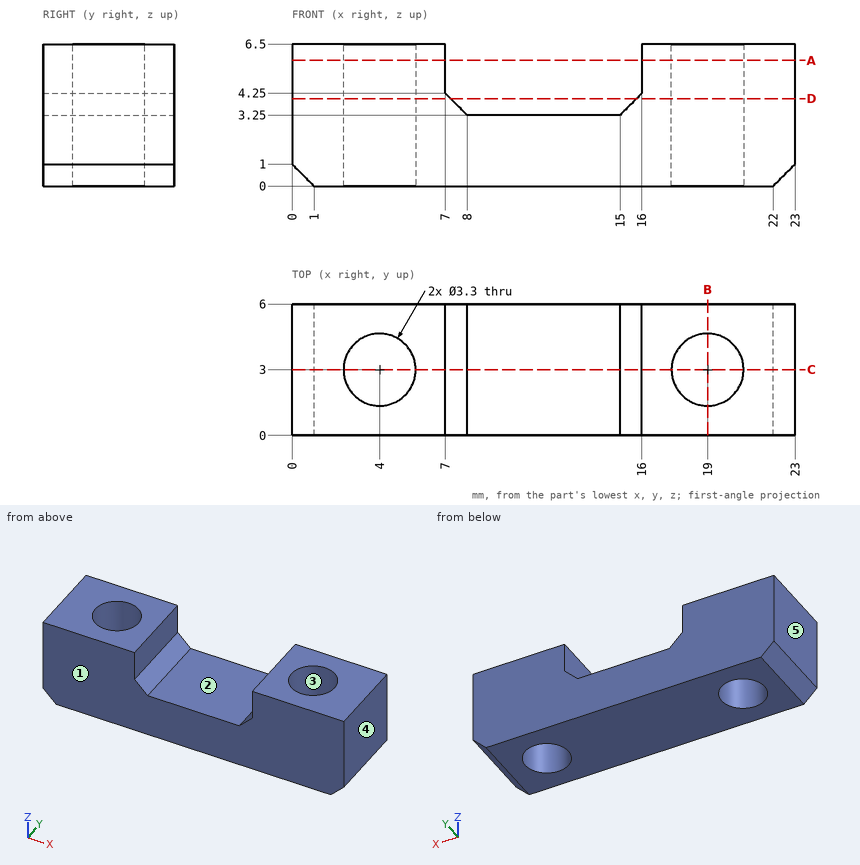
Verification items for this drawing (mm, ordinates from the low corner). A direction names the side the tool comes from. Coordinates: 2 decimals unless noted, no trailing zeros. Loops run counter-clockwise (first coordinate to the right, second up) from the corner with the lowest first, then second, coordinate; pieces in that order, holes last. Notation, with made-up numbers: (-13, -37.75) - (46, -37.75) arc R13 cw to (46, -28.75) - close; hole circle Ø7 at (7, -6.75). An arc over 180 degrees is marked (long way). Use one line per item in the form item = value. Start each with the question number.
Item 1: Gauge pin test, flat end, axial feed: pin 1 (3 mm diameter, centred on x = 11, y = 1.5, fed in from +Z). Record the tip position at first contact, or that the pin passes through.
Item 2: Thickness scan on probe 1 along Y at (x, z) = (4, 3.25); probe 2 along X at (y, z) = (3.55, 1.5); probe 3 along X at (y, z) = (1.8, 3.75). Record the ranges inside material, lowest first.
Item 3: Section check D-D, the plane z = 4. Enter the section's corners in (x, y).
Item 4: Section check B-B, the plane x = 19. Enter the section's corners in (y, z).
Item 5: Tool access check on the marked faces 1 and 2. Record the directions out of +Z, -Z, +X, -X, +Y, -Y that give a thin tool (end or side, any length) a straight path to the whole face; none if there is none.
Item 6: Mould release check, pull along X, two halves, no side actions. Record for the marked faces 3, 4 and 5: +X half, -X half, draft (parallel to the pull), parting line (faces both ways), or undercut.
Item 7: Section check A-A, the plane z = 5.75. Enter the section's corners in (x, y), and give its area (3 significant figures).
Item 8: Section check C-C, the plane y = 3. Enter the section's corners in (x, z), and give its area (4 significant figures).
Computed:
q1.pin_1 = 3.25
q2.probe_1 = 0 to 1.35, 4.65 to 6
q2.probe_2 = 0 to 2.44, 5.56 to 17.44, 20.56 to 23
q2.probe_3 = 0 to 2.87, 5.13 to 7.5, 15.5 to 17.87, 20.13 to 23
q3.outline = (0, 0) - (7.25, 0) - (7.25, 6) - (0, 6) - close; (15.75, 0) - (23, 0) - (23, 6) - (15.75, 6) - close; hole circle Ø3.3 at (4, 3); hole circle Ø3.3 at (19, 3)
q4.outline = (0, 0) - (1.35, 0) - (1.35, 6.5) - (0, 6.5) - close; (4.65, 0) - (6, 0) - (6, 6.5) - (4.65, 6.5) - close
q5.face_1 = +Z, -Z, +X, -X, -Y
q5.face_2 = +Z, +Y, -Y
q6.face_3 = undercut
q6.face_4 = +X half
q6.face_5 = -X half
q7.outline = (0, 0) - (7, 0) - (7, 6) - (0, 6) - close; (16, 0) - (23, 0) - (23, 6) - (16, 6) - close; hole circle Ø3.3 at (4, 3); hole circle Ø3.3 at (19, 3)
q7.area = 66.9 mm2
q8.outline = (0, 1) - (1, 0) - (2.35, 0) - (2.35, 6.5) - (0, 6.5) - close; (5.65, 0) - (17.35, 0) - (17.35, 6.5) - (16, 6.5) - (16, 4.25) - (15, 3.25) - (8, 3.25) - (7, 4.25) - (7, 6.5) - (5.65, 6.5) - close; (20.65, 0) - (22, 0) - (23, 1) - (23, 6.5) - (20.65, 6.5) - close
q8.area = 77.35 mm2
